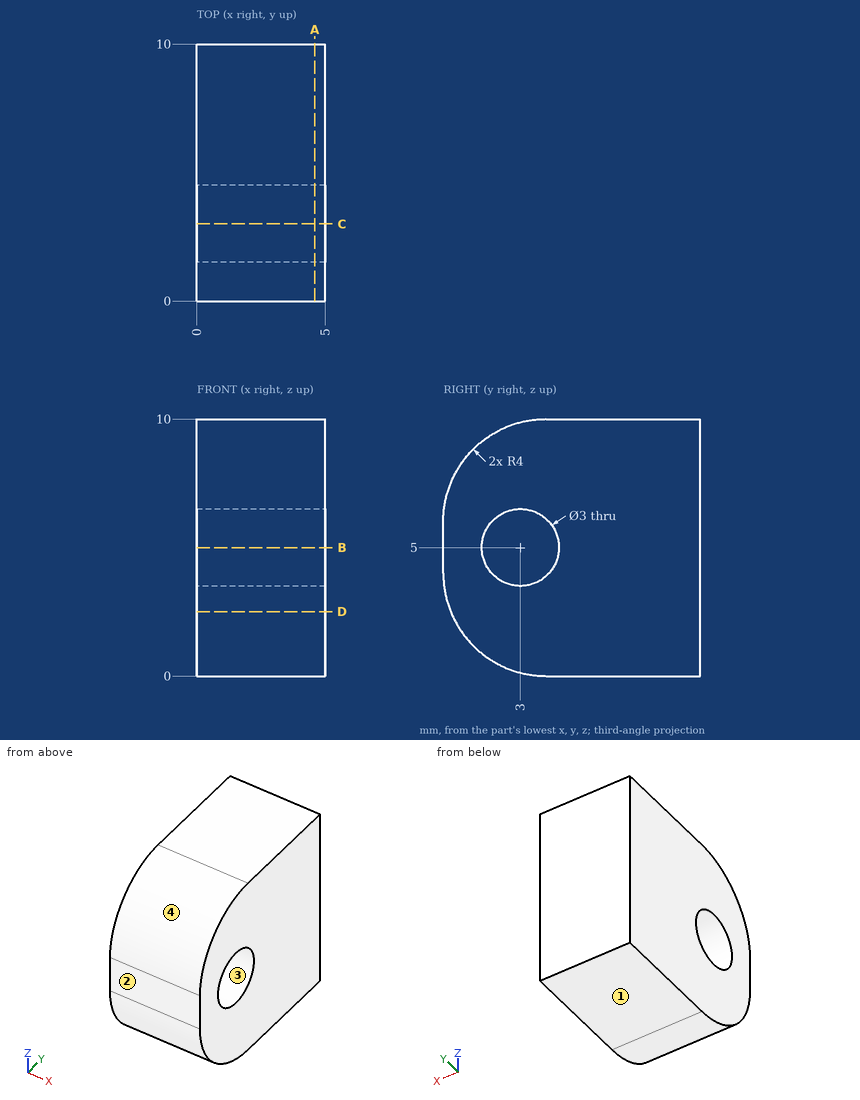
Drawing for the job (mm, zero at the part's lowest x, y, z). Give positions to 0.01 mm unless a question says otherwise; leave off trailing zeros. Loops run counter-clockwise (first coordinate to the right, second up) from the corner with the lowest first, then second, coordinate; pieces in that order, holes last.
(1) Band-saw the part on D-D (z = 2.5). Write the cut outline in (x, y).
Return value:
outline: (0, 0.29) - (5, 0.29) - (5, 10) - (0, 10) - close
(2) Pull direction Z, two halves, no side cores. Call the marked faces 1, 2, 3 and 4: pulls with the +Z half, pulls with the -Z half, needs draft (parallel to the pull), parting line crosses it, or undercut.
Return value:
face 1: pulls with the -Z half
face 2: needs draft
face 3: undercut
face 4: pulls with the +Z half
(3) Band-saw the part on A-A (x = 4.6). Write the cut outline in (y, z).
Return value:
outline: (0, 4) arc R4 ccw to (4, 0) - (10, 0) - (10, 10) - (4, 10) arc R4 ccw to (0, 6) - close; hole circle Ø3 at (3, 5)
(4) Drill centre lines: line 1 along Y through (x, z) = (4, 5); line 2 along Y through (x, z) = (1.1, 3.75); line 3 along Z through (x, y) = (2.15, 3.5). Where is each one in solid material? Low to high.
Return value:
line 1: y = 0 to 1.5, 4.5 to 10
line 2: y = 0.01 to 2.17, 3.83 to 10
line 3: z = 0.03 to 3.59, 6.41 to 9.97
(5) Band-saw the part on B-B (z = 5). Write the cut outline in (x, y).
Return value:
outline: (0, 0) - (5, 0) - (5, 1.5) - (0, 1.5) - close; (0, 4.5) - (5, 4.5) - (5, 10) - (0, 10) - close
(6) Pin check, flat tip, straight feed: pin 1 (2.5 mm diameter, centred on y = 3, z = 5, fed in from -X). Stop position of the tip, or through.
Return value:
pin 1: passes through
(7) Band-saw the part on C-C (y = 3). Write the cut outline in (x, z), and give its area (3 significant figures).
Return value:
outline: (0, 0.13) - (5, 0.13) - (5, 3.5) - (0, 3.5) - close; (0, 6.5) - (5, 6.5) - (5, 9.87) - (0, 9.87) - close
area: 33.7 mm2
